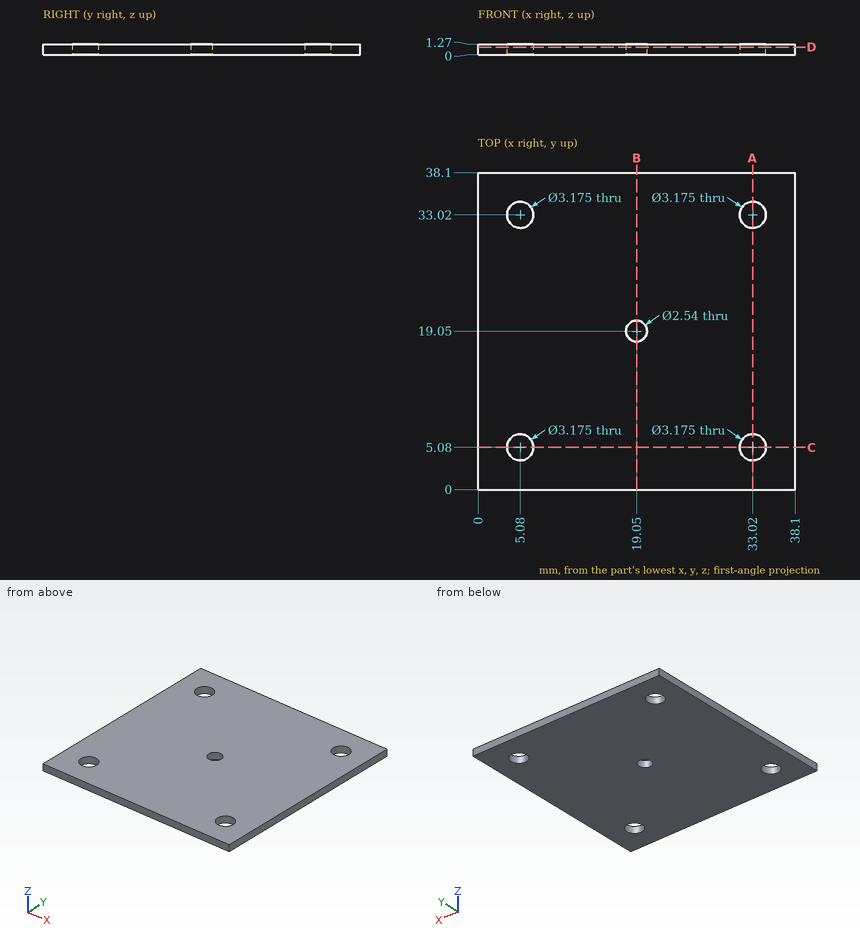
Verification items for this drawing (mm, ordinates from the low corner). Coordinates: 2 decimals unless noted, no trailing zeros. Order: outer loops, then holes, each group sorted by start corner. A loop starts at its lowest first (then second) coordinate and runs counter-clockwise, first axis right, second up. Notation, with made-up numbers: (63.25, -31) - (74.25, -31) arc R20 ccw to (74.25, -8) - close; hole circle Ø7 at (-38.5, -15.5). An arc over 180 degrees is marked (long way). Answer as a JSON object with one key per item and string values. Group by question number.
Item 1: Depth check by flat-ended pin: pin 1 Ø3 at (x, y) = (33.02, 33.02) entering from -Z. Enter the tip coordinate at first touch or a pass-through.
Item 2: Sectioned sample at B-B, the plane x = 19.05. Record the cut outline in (y, z).
Item 3: Sectioned sample at A-A, the plane x = 33.02. Record the cut outline in (y, z), and give its area (3 significant figures).
Item 4: Scan lines: probe 1 along X at (y, z) = (5.08, 0.45); probe 2 along Y at (x, z) = (4, 0.75). Record each from-to range of solid material in increasing order.
Item 5: Sectioned sample at D-D, the plane z = 0.9. Give the number of separate pieces and of enclosed holes in the cut face, and give its area (3 significant figures).
Resolved:
{
 "1": {"pin 1": "through"},
 "2": {"outline": "(0, 0) - (17.78, 0) - (17.78, 1.27) - (0, 1.27) - close; (20.32, 0) - (38.1, 0) - (38.1, 1.27) - (20.32, 1.27) - close"},
 "3": {"outline": "(0, 0) - (3.49, 0) - (3.49, 1.27) - (0, 1.27) - close; (6.67, 0) - (31.43, 0) - (31.43, 1.27) - (6.67, 1.27) - close; (34.61, 0) - (38.1, 0) - (38.1, 1.27) - (34.61, 1.27) - close", "area": "40.3 mm^2"},
 "4": {"probe 1": "0 to 3.49, 6.67 to 31.43, 34.61 to 38.1", "probe 2": "0 to 3.92, 6.24 to 31.86, 34.18 to 38.1"},
 "5": {"separate pieces": "1", "enclosed holes": "5", "area": "1,410 mm^2"}
}
